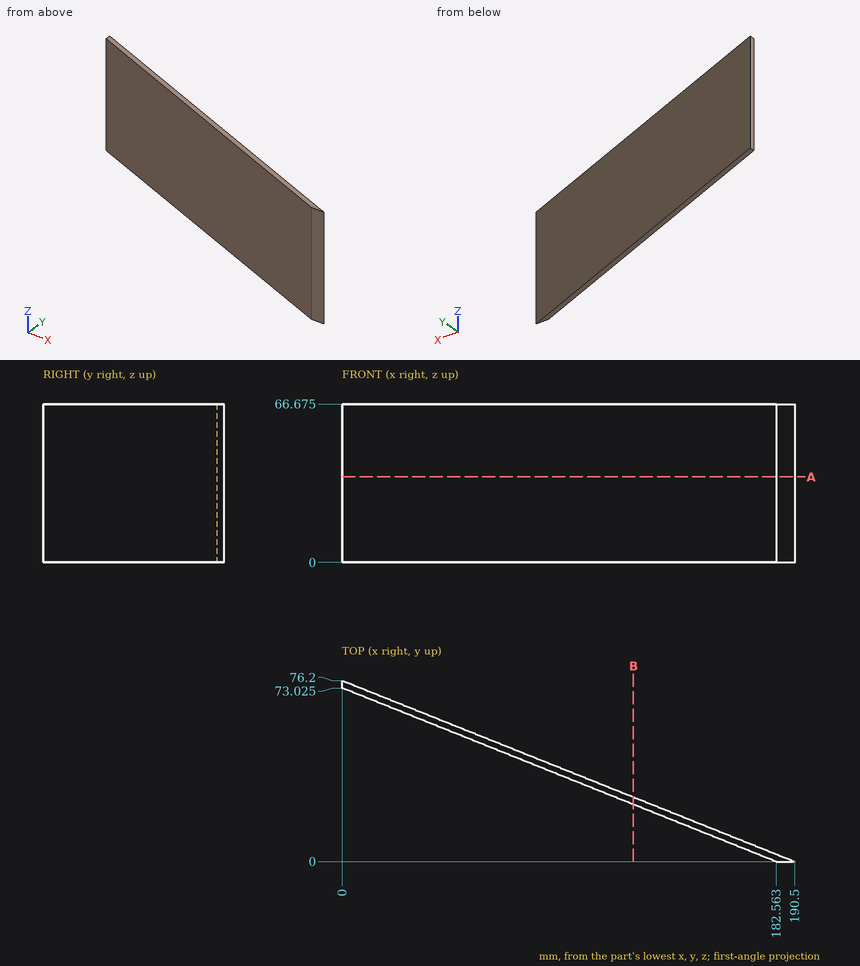
Geometry: see drawing. Coordinates: mm, zero at the bounding-box minimum. Give positions to 0.01 mm unless a question says otherwise; leave off trailing zeros. Loops run counter-clockwise (first coordinate to the right, second up) from the corner with the lowest first, then second, coordinate; pieces in that order, holes last. Notation, with made-up numbers: (3.25, 0) -> (12.25, 0) arc R15 ccw to (12.25, 18) -> close; hole circle Ø9 at (56, 46). An arc over 180 degrees is marked (long way). Put each result on its own line as item: value.
1. Cut plane A-A (z = 36). Return the cut outline in (x, y) (1 decimal).
Taken from the geometry:
outline: (0, 73) -> (182.6, 0) -> (190.5, 0) -> (0, 76.2) -> close
2. Pin query (flat end, axial travel): P1, Ø1.5, axis at x = 80, z = 24.5, coming from the -Y side (1 decimal); P2, Ø1, axis at x = 78, z = 22, coming from the -Y side (1 decimal); P3, Ø2, axis at y = 10, z = 60, coming from the -X side (1 decimal). Return the tip coordinate at first contact, or that it passes through.
Taken from the geometry:
P1: stops at y = 40.7
P2: stops at y = 41.6
P3: stops at x = 155.1
3. Cut plane B-B (x = 122.5). Return the cut outline in (y, z) (1 decimal), plus the area to 3 significant figures.
Taken from the geometry:
outline: (24, 0) -> (27.2, 0) -> (27.2, 66.7) -> (24, 66.7) -> close
area: 212 mm2
4. Ray query, line 1 along Y through (x, z) = (31, 29) (1 decimal); line 2 along Y through (x, z) = (95, 22) (1 decimal). Return the intervals inside material, ascending. Write a range as [from, to].
Taken from the geometry:
line 1: y = [60.6, 63.8]
line 2: y = [35, 38.2]
